```python
from build123d import *

# Parameters (mm, degrees)
F0_R          = 28.375
F0_R_2        = 24
F1_DEPTH      = 65
F3_DEPTH      = 35
F3_DEPTH_BACK = 35
F5_DEPTH      = 35
F7_DEPTH      = 5
F9_DEPTH      = 25
F11_R         = 24
F11_R_2       = 21
F12_DEPTH     = 3


with BuildPart() as f1:
    # F0 (on Front) → F1 (new body)
    with BuildSketch(Plane.XZ):
        Circle(F0_R)
        Circle(F0_R_2, mode=Mode.SUBTRACT)
    extrude(amount=F1_DEPTH)

    # F2 (on Right) → F3 (cut, two sides)
    with BuildSketch(Plane.YZ) as f3_sk:
        Polygon((-55, -28.75), (-65, 28.75), (-65, -28.75), align=None)
    extrude(amount=F3_DEPTH, mode=Mode.SUBTRACT)
    extrude(f3_sk.sketch, amount=-F3_DEPTH_BACK, mode=Mode.SUBTRACT)

    # F4 (on Top) → F5 (cut)
    with BuildSketch(Plane.XY):
        with BuildLine():
            Line((5.25, 0), (-5, 0))
            Line((-5, 0), (-5, -26.5))
            ThreePointArc((-5, -26.5), (-4.12132, -28.62132), (-2, -29.5))
            Line((-2, -29.5), (2.25, -29.5))
            ThreePointArc((2.25, -29.5), (4.37132, -28.62132), (5.25, -26.5))
            Line((5.25, -26.5), (5.25, 0))
        make_face()
    extrude(amount=-F5_DEPTH, mode=Mode.SUBTRACT)

    # F6 (on Front) → F7 (join)
    with BuildSketch(Plane.XZ):
        with BuildLine():
            Line((11.5, 11.5), (11.5, -25.529395))
            ThreePointArc((11.5, -25.529395), (0, 28), (-11.5, -25.529395))
            Line((-11.5, -25.529395), (-11.5, 11.5))
            ThreePointArc((-11.5, 11.5), (0, 23), (11.5, 11.5))
        make_face()
    extrude(amount=F7_DEPTH)

    # F8 (on face) → F9 (cut)
    with BuildSketch(Plane(origin=(0, 0, 0), x_dir=(-1, 0, 0), z_dir=(0, 1, 0))):
        with BuildLine():
            Line((-17, -2.75), (-10, -2.75))
            ThreePointArc((-10, -2.75), (-7.25, 0), (-10, 2.75))
            Line((-10, 2.75), (-17, 2.75))
            ThreePointArc((-17, 2.75), (-19.75, 0), (-17, -2.75))
        make_face()
        with BuildLine():
            Line((17, 2.75), (10, 2.75))
            ThreePointArc((10, 2.75), (7.25, 0), (10, -2.75))
            Line((10, -2.75), (17, -2.75))
            ThreePointArc((17, -2.75), (19.75, 0), (17, 2.75))
        make_face()
    extrude(amount=-F9_DEPTH, mode=Mode.SUBTRACT)

    # F11 (on offset) → F12 (join)
    with BuildSketch(Plane.XZ.offset(45)):
        Circle(F11_R)
        Circle(F11_R_2, mode=Mode.SUBTRACT)
    extrude(amount=F12_DEPTH)


solid = f1.part
```
Geometry check sheet. Reference: the model listing, model coordinates, mm. A direction names the side the tool comes from. Coordinates: 2 decimals unless noted, no trailing zeros. Loops run counter-clockwise (first coordinate to the right, second up) from the corner with the lowest first, then second, coordinate; pieces in that order, holes last.
Item 1: Access from +Z, -Z, +X, -X, +Y, -Y to the whole of each face (thin tool, end or side, straight path). Record for faces 1 (the face through (-3.1, -54.2, 23.8)), 2 (the face through (-0.1, -45, -21.2)), 3 (the face through (14, -2, 2.75)), 4 (the face through (-11.5, -2, -12)).
Item 2: Go/stop test with flat-tipped pins: pin 1 Ø12 at (y, z) = (-39, -2) entering from -X (3 decimals); pin 2 Ø3.5 at (y, z) = (-19, -25.5) entering from +X; pin 3 Ø2.5 at (y, z) = (-2, 6.5) entering from +X; pin 4 Ø8 at (x, y) = (-8.5, -41.5) entering from +Z. Record where each tip stops, or that it passes through.
Item 3: Sectioned sample at B-B, the plane z = -4. Record the boundary of the cut face in (x, y), then the cut area to 3 significant figures.
Item 4: Release check for a two-part mould opening along Z. For faces 5 (the face through (-3.694, -32.013, 28.134)), 6 (the face through (-14, -2, 2.75)), 7 (the face through (12, 0, -6)) record: released by +Z, released by -Z, zero draft, split by the parting line, or undercut.
Item 5: Thickness scan on line 1 (X direction, y = -16, z = 0) (3 decimals); line 2 (Z direction, x = 0, y = -47) (3 decimals). Record the ranges inside material, lowest first.
Item 6: Sectioned sample at A-A, the plane x = 6.5. Record the boundary of the cut face in (y, z).
Item 7: Sectioned sample at C-C, the plane y = -33. Record the boundary of the cut face in (x, z) (3 decimals), then the cut area to 3 significant figures.
Item 8: Sectioned sample at D-D, the plane y = -10. Record the boundary of the cut face in (x, z) (3 decimals), then the cut area to 3 significant figures.
Check result:
1. face 1: -Y
1. face 2: none
1. face 3: +Y, -Y
1. face 4: +Y
2. pin 1: stops at x = -28.375
2. pin 2: stops at x = 15.53
2. pin 3: stops at x = 27.89
2. pin 4: stops at z = 28.02
3. outline: (-28.09, -59.3) - (-23.66, -59.3) - (-23.66, -48) - (-20.62, -48) - (-20.62, -45) - (-23.66, -45) - (-23.66, -5) - (-11.5, -5) - (-11.5, 0) - (-28.09, 0) - close; (11.5, -5) - (23.66, -5) - (23.66, -45) - (20.62, -45) - (20.62, -48) - (23.66, -48) - (23.66, -59.3) - (28.09, -59.3) - (28.09, 0) - (11.5, 0) - close
3. area: 665 mm2
4. face 5: split by the parting line
4. face 6: undercut
4. face 7: zero draft
5. line 1: x = -28.375 to -24, 24 to 28.375
5. line 2: z = -28.375 to -21, 21 to 28.375
6. outline: (-64.8, 27.62) - (-64.02, 23.1) - (-48, 23.1) - (-48, 19.97) - (-45, 19.97) - (-45, 23.1) - (-5, 23.1) - (-5, 20.99) - (0, 20.99) - (0, 27.62) - close; (-55.98, -23.1) - (-55.2, -27.62) - (0, -27.62) - (0, -23.1) - (-45, -23.1) - (-45, -19.97) - (-48, -19.97) - (-48, -23.1) - close
7. outline: circle Ø56.75 at (0, 0); hole circle Ø48 at (0, 0)
7. area: 720 mm2
8. outline: (-5, -27.931) - (-5, -23.473) arc R24 cw (long way) to (5.25, -23.419) - (5.25, -27.885) arc R28.375 ccw (long way) to start
8. area: 675 mm2
